The model under review builds one solid part; all positions refer to its coordinate system, in mm. A direction names the side the tool comes from. Round coordinates to 2 decimals unless told otherwise and drop trailing zeros. Order: outer loops, then holes, each group sorted by start corner. A loop starts at its lowest first (then second) coordinate and runs counter-clockwise, first axis right, second up. Notation, with made-up numbers: (-4, 73) -> (11, 73) arc R22 ccw to (11, 90) -> close; hole circle Ø8 at (-29.5, 9). An arc over 180 degrees is marked (long way). Use a Markdown table: item, result. Add a question column.
```python
from build123d import *

# Parameters (mm, degrees)
SKETCH007_R      = 4.125
EXTRUDE009_DEPTH = 4
EXTRUDE008_DEPTH = 44


with BuildPart() as extrude009:
    # Sketch007 → Extrude009 (new body)
    with BuildSketch(Plane.XZ):
        Polygon((-24, 98), (-20, 98), (20, 98), (24, 98), (122, 0), (118, 0), (78, 0), (74, 0), (4, 70), (-4, 70), (-74, 0), (-78, 0), (-118, 0), (-122, 0), align=None)
        with Locations((0, 78.125)):
            Circle(SKETCH007_R, mode=Mode.SUBTRACT)
    extrude(amount=EXTRUDE009_DEPTH)


with BuildPart() as stage_2_paths:
    # Sketch006 → Extrude008 (new body)
    with BuildSketch(Plane.XZ):
        Polygon((-20, 98), (-118, 0), (-120, 1.154701), (-122, 0), (-24, 98), (-22, 99.154701), align=None)
        Polygon((118, 0), (20, 98), (22, 99.154701), (24, 98), (122, 0), (120, 1.154701), align=None)
        Polygon((-4, 70), (-74, 0), (-76, 1.154701), (-78, 0), (-4, 74), (4, 74), (78, 0), (76, 1.154701), (74, 0), (4, 70), align=None)
    extrude(amount=EXTRUDE008_DEPTH)


with BuildPart() as stage_2_paths_1:
    # Extrude008 placement: moved
    add(stage_2_paths.part.moved(Location((0, -4, 0))))

    # Fusion002: union Extrude009
    add(extrude009.part)


solid = stage_2_paths_1.part
```
Q1. To check wall thickness, follow line 1 along Z through (x, y) = (0, -3); line 2 along X through (y, z) = (-16, 18.5); line 3 along X through (y, z) = (-12, 73). State the ranges of each line that lie inside material, in increasing order.
Q2. Add section C-C, the plane x = -43. Give the boundary of the cut face in (y, z).
Q3. For faces 1 (the face through (-17, -48, 59)), 2 (the face through (-39, -24, 35)), 3 (the face through (40, -26, 38)), list the 3-axis set-ups (+Z, -Z, +X, -X, +Y, -Y) from which the entire face can be reached by the end or side of a thin tool; tool diameter is ignored.
Q4. Add section B-B, the plane y = -29. Give the boundary of the cut face in (x, z), then the cut area to 3 significant figures.
Q5. Add section D-D, the plane z = 86.5. Give the boundary of the cut face in (x, y), then the cut area to 3 significant figures.
Q6. Draft analysis for pull direction X (two halves, no side actions). For faces 4 (the face through (72, -24, 50)), 5 (the face through (-74, -24, 48)), 6 (the face through (-75, -48, 46)), 7 (the face through (0, -26, 74)), state which applies: released by +X, released by -X, zero draft, split by the parting line, or undercut.
Q7. For pin 1 (2 mm diameter, centred on x = 94, y = -9.5, fed in from -Z); pin 2 (3 mm diameter, centred on x = -4, z = 78, fed in from -Y); pin 3 (1 mm diameter, centred on x = -16.5, y = -39.5, fed in from -Z), all flat-tipped, find the tip position at first contact; note any pin that passes through.
Q8. Add section A-A, the plane z = 62. Give the boundary of the cut face in (x, y).
Return value:
| question | item | result |
|---|---|---|
| 1 | line 1 | 70 to 74, 82.25 to 98 |
| 1 | line 2 | -103.5 to -99.5, -59.5 to -55.5, 55.5 to 59.5, 99.5 to 103.5 |
| 1 | line 3 | -49 to -45, -5 to 5, 45 to 49 |
| 2 | outline | (-48, 31) -> (0, 31) -> (0, 79) -> (-48, 79) -> (-48, 75) -> (-4, 75) -> (-4, 35) -> (-48, 35) -> close |
| 3 | face 1 | +Z, -Z, +X, -X, -Y |
| 3 | face 2 | -Z, +Y, -Y |
| 3 | face 3 | -Y |
| 4 | outline | (-122, 0) -> (-120, 1.15) -> (-118, 0) -> (-20, 98) -> (-22, 99.15) -> (-24, 98) -> close; (-78, 0) -> (-76, 1.15) -> (-74, 0) -> (-4, 70) -> (4, 70) -> (74, 0) -> (76, 1.15) -> (78, 0) -> (4, 74) -> (-4, 74) -> close; (20, 98) -> (118, 0) -> (120, 1.15) -> (122, 0) -> (24, 98) -> (22, 99.15) -> close |
| 4 | area | 1,390 mm² |
| 5 | outline | (-35.5, -48) -> (-31.5, -48) -> (-31.5, -4) -> (31.5, -4) -> (31.5, -48) -> (35.5, -48) -> (35.5, 0) -> (-35.5, 0) -> close |
| 5 | area | 636 mm² |
| 6 | face 4 | released by +X |
| 6 | face 5 | released by -X |
| 6 | face 6 | zero draft |
| 6 | face 7 | undercut |
| 7 | pin 1 | z = 23 |
| 7 | pin 2 | y = -4 |
| 7 | pin 3 | z = 57 |
| 8 | outline | (-60, -48) -> (-56, -48) -> (-56, -4) -> (-16, -4) -> (-16, -48) -> (-12, -48) -> (-12, 0) -> (-60, 0) -> close; (12, -48) -> (16, -48) -> (16, -4) -> (56, -4) -> (56, -48) -> (60, -48) -> (60, 0) -> (12, 0) -> close |
